from build123d import *

# Parameters (mm, degrees)
CHAMFER_1_SIZE      = 1
FILLET_1_R          = 0.4
SKETCH_2_R          = 1.5
CUT_EXTRUDE_1_DEPTH = 6.8
CHAMFER_2_SIZE      = 0.2
CHAMFER_2_SIZE_2    = 0.196621941


with BuildPart() as part:
    # 스케치1 → 회전1 (revolve)
    with BuildSketch(Plane(origin=(0, 0, 0), x_dir=(1, 0, 0), z_dir=(0, 1, 0))):
        with BuildLine():
            Line((0, 0), (4, 0))
            Line((4, 0), (5.894700278586023, 2))
            Line((5.894700278586023, 2), (9.7, 2))
            Line((9.7, 2), (9.7, -10))
            Line((9.7, -10), (8.2, -9.999999999999998))
            Line((8.2, -9.999999999999998), (7.5, -2.999999999999999))
            ThreePointArc((7.5, -2.999999999999999), (3.75282938430565, -3.220734607641745), (0, -3.3))
            Line((0, -3.3), (0, -3))
            Line((0, -3), (0, 0))
        make_face()
    revolve(axis=Axis((0, 0, 3), (0, 0, -1)))

    # 모따기1
    chamfer_1_edges = [part.edges().sort_by_distance(p)[0] for p in [
        (-9.7, -1.19e-15, 10),
        (-9.7, -1.19e-15, -2),
    ]]
    chamfer(chamfer_1_edges, length=CHAMFER_1_SIZE)

    # 필렛1
    fillet_1_edges = [part.edges().sort_by_distance(p)[0] for p in [
        (-8.2, -1e-15, 9.999999999999998),
        (-5.894700278586023, -7.2e-16, -2),
    ]]
    fillet(fillet_1_edges, radius=FILLET_1_R)

    # 스케치2 → 컷-돌출1 (cut)
    with BuildSketch(Plane.XY.offset(10)):
        Circle(SKETCH_2_R)
    extrude(amount=-CUT_EXTRUDE_1_DEPTH, mode=Mode.SUBTRACT)

    # 모따기2
    # the kernel refuses this chamfer: 0.2, 0.196621941 mm, written as the material it takes off along each edge
    with BuildSketch(Plane(origin=(2.26883e-11, 1.9670789e-10, 3.2853073545034164), x_dir=(1.0, -1.3113829668845467e-10, 0), z_dir=(-1.3113829668845467e-10, -1.0, 0))) as chamfer_2_piece_1_section:
        with BuildLine():
            Line((1.499999999977312 + CHAMFER_2_SIZE * 0.999831893416, -CHAMFER_2_SIZE * 0.0183353458825), (1.5000000000226883, -CHAMFER_2_SIZE_2 * 1.00000000195))
            Line((1.5000000000226883, -CHAMFER_2_SIZE_2 * 1.00000000195), (1.499999999977312, 0))
            ThreePointArc((1.499999999977312, 0), (1.6028105859636501, -0.00183517420042278), (1.499999999977312 + CHAMFER_2_SIZE * 0.999831893416, -CHAMFER_2_SIZE * 0.0183353458825))
        make_face()
    chamfer_2_piece_1 = revolve(axis=Axis((2.26883e-11, 1.9670789e-10, 3.2853073545034164), (0, 0, 1)), mode=Mode.PRIVATE)
    chamfer_2_piece_1 = split(chamfer_2_piece_1, bisect_by=Plane(origin=(2.26883e-11, 1.9670789e-10, 3.2), z_dir=(0, 0, 1)), keep=Keep.TOP, mode=Mode.PRIVATE)
    add(chamfer_2_piece_1, mode=Mode.SUBTRACT)


solid = part.part
Check sheet for the modelled part. Datum: model origin and axes. Units: mm. A direction names the side the tool comes from. Round coordinates to 2 decimals unless told otherwise and drop trailing zeros. Loops run counter-clockwise (first coordinate to the right, second up) from the corner with the lowest first, then second, coordinate; pieces in that order, holes last. Notation, with made-up numbers: (4, 22) -> (49, 22) arc R7 ccw to (49, 26) -> close; hole circle Ø2 at (-10.75, 47.5). An arc over 180 degrees is marked (long way). Put each result on its own line as item: value. Start each with the question number.
1. Scan lines: probe 1 along Z at (x, y) = (0.5, -1.5); probe 2 along Y at (x, z) = (-1.75, 4.5); probe 3 along Y at (x, z) = (5, 5.5). Record each from-to range of solid material in increasing order.
2. Section check A-A (z = 5). Enter the section's corners in (x, y).
3. Section check B-B (z = 0.5). Enter the section's corners in (x, y), plus the area to 3 significant figures.
4. Access from +Z, -Z, +X, -X, +Y, -Y to the whole of each face (thin tool, end or side, straight path). Record for faces 1 (the face through (0, 0, 0)), 2 (the face through (-7.746, -0.341, 5.536)).
5. Draft check along Y on faces 3 (the face through (-2, -6, -2)), 4 (the face through (0, 0, 3.2)), 5 (the face through (3.921, -1.235, -0.117)), 6 (the face through (9.252, -2.914, 4.07)). Enter one of: +Y half, -Y half, draft (parallel to the pull), parting line (faces both ways), or undercut.
6. Section check C-C (z = 7.25). Enter the section's corners in (x, y) (3 decimals), plus the area to 3 significant figures.
7. Gauge pin test, flat ends, axial feed: pin 1 (2 mm diameter, centred on x = -4, z = 5, fed in from -Y); pin 2 (2 mm diameter, centred on x = -5.5, z = 9, fed in from +Y); pin 3 (2.5 mm diameter, centred on x = -1, y = 0.5, fed in from -Z). Record the tip position at first contact, or that the pin passes through.
Findings:
1. probe 1: z = 0 to 3.2
1. probe 2: y = -9.54 to -7.45, 7.45 to 9.54
1. probe 3: y = -8.31 to -5.92, 5.92 to 8.31
2. outline: circle Ø19.4 at (0, 0); hole circle Ø15.4 at (0, 0)
3. outline: circle Ø19.4 at (0, 0)
3. area: 296 mm^2
4. face 1: -Z
4. face 2: +Z
5. face 3: draft
5. face 4: undercut
5. face 5: undercut
5. face 6: parting line
6. outline: circle Ø19.4 at (0, 0); hole circle Ø15.85 at (0, 0)
6. area: 98.3 mm^2
7. pin 1: stops at y = -9.22
7. pin 2: stops at y = 8.59
7. pin 3: stops at z = 0
